Geometry check sheet. Reference: the model listing, model coordinates, mm. A direction names the side the tool comes from. Round coordinates to 2 decimals unless told otherwise and drop trailing zeros. Order: outer loops, then holes, each group sorted by start corner. A loop starts at its lowest first (then second) coordinate and runs counter-clockwise, first axis right, second up. Notation, with made-up numbers: (76, 77.25) - (117, 77.25) arc R28 ccw to (117, 98.25) - close; hole circle Ø1 at (80.5, -28). An arc over 180 degrees is marked (long way). One line per question, with ' | ' between items. Start each with the question number.
Q1. Sectioned sample at A-A, the plane z = 3.25. Enter the section's corners in (x, y), then the cut area to 3 significant figures.
Q2. Sectioned sample at D-D, the plane z = 4.75. Enter the section's corners in (x, y), then the cut area to 3 significant figures.
Q3. Gauge pin test, flat ends, axial feed: P1, Ø6, axis at x = 6.5, y = 0, coming from the +Z side; P2, Ø3, axis at y = 3.5, z = 2, coming from the -X side; P3, Ø1, axis at x = 1.5, y = -4, coming from the +Z side; P4, Ø2.5, axis at x = -6.4, y = 0, coming from the -Z side. Record the tip position at first contact, or that the pin passes through.
Q4. Tool access check on faces 1 (the face through (0, -5.2, 2)), 2 (the face through (-1, -3.7, 6)), 3 (the face through (-2.746, -4, 5)), 4 (the face through (4, -4, 3.9)), 5 (the face through (10.1, 0.1, 2)). Record the directions out of +Z, -Z, +X, -X, +Y, -Y that give a thin tool (end or side, any length) a straight path to the whole face; none if there is none.
Q5. Sectioned sample at C-C, the plane x = 3. Enter the section's corners in (y, z), then the cut area to 3 significant figures.
Q6. Material ranges on line 1 along Y through (x, z) = (-6.4, 3.6); line 2 along Y through (x, z) = (6.4, 0.8); line 3 along Z through (x, y) = (-0.5, -4.25), recorded low to high.
Q7. Sectioned sample at B-B, the plane y = 0. Enter the section's corners in (x, z).
Q8. Mould release check, pull along Y, two halves, no side actions. Record for faces 6 (the face through (-4.746, 4, 5)), 7 (the face through (11.6, -0.1, 1.2)), 8 (the face through (3, 0, 1.5)): +Y half, -Y half, draft (parallel to the pull), parting line (faces both ways), or undercut.
```python
from build123d import *

# Parameters (mm, degrees)
F1_DEPTH  = 1.5
F3_DEPTH  = 4
F4_DEPTH  = 1
F6_DEPTH  = 2.6
F7_R      = 1.6
F7_R_2    = 2.75
F8_DEPTH  = 1.501
F10_DEPTH = 5
F11_W     = 2
F11_H     = 1.5
F12_DEPTH = 1.4
F13_W     = 2
F13_H     = 1.5
F14_DEPTH = 1.4


with BuildPart() as f1:
    # F0 (on Top) → F1 (new body)
    with BuildSketch(Plane.XY):
        with BuildLine():
            Line((6.4, 5.2), (-6.4, 5.2))
            ThreePointArc((-6.4, 5.2), (-11.6, 0), (-6.4, -5.2))
            Line((-6.4, -5.2), (6.4, -5.2))
            ThreePointArc((6.4, -5.2), (11.6, 0), (6.4, 5.2))
        make_face()
    extrude(amount=F1_DEPTH)

    # F2 (on face) → F3 (join)
    with BuildSketch(Plane.XY.offset(1.5)):
        with BuildLine():
            Line((0, 5.2), (-6.4, 5.2))
            ThreePointArc((-6.4, 5.2), (-11.6, 0), (-6.4, -5.2))
            Line((-6.4, -5.2), (0, -5.2))
            Line((0, -5.2), (0, -3.7))
            Line((0, -3.7), (-6.4, -3.7))
            ThreePointArc((-6.4, -3.7), (-10.1, 0), (-6.4, 3.7))
            Line((-6.4, 3.7), (0, 3.7))
            Line((0, 3.7), (0, 5.2))
        make_face()
    extrude(amount=F3_DEPTH)

    # F2 (on face) → F4 (join)
    with BuildSketch(Plane.XY.offset(1.5)):
        with BuildLine():
            Line((6.4, 5.2), (0, 5.2))
            Line((0, 5.2), (0, 3.7))
            Line((0, 3.7), (6.4, 3.7))
            ThreePointArc((6.4, 3.7), (10.1, 0), (6.4, -3.7))
            Line((6.4, -3.7), (0, -3.7))
            Line((0, -3.7), (0, -5.2))
            Line((0, -5.2), (6.4, -5.2))
            ThreePointArc((6.4, -5.2), (11.6, 0), (6.4, 5.2))
        make_face()
    extrude(amount=F4_DEPTH)

    # F5 (on face) → F6 (join)
    with BuildSketch(Plane.XY.offset(1.5)):
        with BuildLine():
            Line((-6.4, -3.7), (-2.746235, -3.7))
            ThreePointArc((-2.746235, -3.7), (-1.2, 0), (-2.746235, 3.7))
            Line((-2.746235, 3.7), (-6.4, 3.7))
            ThreePointArc((-6.4, 3.7), (-2.7, 0), (-6.4, -3.7))
        make_face()
    extrude(amount=F6_DEPTH)

    # F7 (on face) → F8 (cut, through all)
    with BuildSketch(Plane.XY.offset(1.5)):
        with Locations((-6.4, 0)):
            Circle(F7_R)
        with Locations((6.4, 0)):
            Circle(F7_R_2)
    extrude(amount=-F8_DEPTH, mode=Mode.SUBTRACT)

    # F9 (on face) → F10 (join)
    with BuildSketch(Plane.XY.offset(1.5)):
        with BuildLine():
            Line((-2.746235, -3.7), (0, -3.7))
            Line((0, -3.7), (0, 3.7))
            Line((0, 3.7), (-2.746235, 3.7))
            ThreePointArc((-2.746235, 3.7), (-1.2, 0), (-2.746235, -3.7))
        make_face()
    extrude(amount=F10_DEPTH)

    # F11 (on face) → F12 (cut, through all)
    with BuildSketch(Plane.XY.offset(5.5)):
        with Locations((-3.746235, -4.45)):
            Rectangle(F11_W, F11_H)
        with Locations((-3.746235, 4.45)):
            Rectangle(F11_W, F11_H)
    extrude(amount=-F12_DEPTH, mode=Mode.SUBTRACT)

    # F13 (on face) → F14 (join)
    with BuildSketch(Plane.XY.offset(2.5)):
        with Locations((3.746235, -4.45)):
            Rectangle(F13_W, F13_H)
    extrude(amount=F14_DEPTH)


solid = f1.part
```
Determined:
1) outline: (-6.4, -5.2) - (0, -5.2) - (0, 5.2) - (-6.4, 5.2) arc R5.2 ccw to start; (2.75, -5.2) - (4.75, -5.2) - (4.75, -3.7) - (2.75, -3.7) - close; hole circle Ø7.4 at (-6.4, 0) | area: 69.0 mm2
2) outline: (-6.4, -5.2) - (-4.75, -5.2) - (-4.75, -3.7) - (-6.4, -3.7) arc R3.7 cw to (-6.4, 3.7) - (-4.75, 3.7) - (-4.75, 5.2) - (-6.4, 5.2) arc R5.2 ccw to start; (-2.75, -5.2) - (0, -5.2) - (0, 5.2) - (-2.75, 5.2) - (-2.75, 3.7) arc R5.2 cw to (-2.75, -3.7) - close | area: 46.6 mm2
3) P1: stops at z = 1.5 | P2: stops at x = -11.2 | P3: stops at z = 2.5 | P4: passes through
4) face 1: +Z, -Z, +X, -X, -Y | face 2: +Z, +X, -X, -Y | face 3: +Z, +Y, -Y | face 4: +Z, +X, +Y, -Y | face 5: +Z
5) outline: (-5.2, 0) - (5.2, 0) - (5.2, 2.5) - (3.7, 2.5) - (3.7, 1.5) - (-3.7, 1.5) - (-3.7, 3.9) - (-5.2, 3.9) - close | area: 20.7 mm2
6) line 1: y = -5.2 to -3.7, 3.7 to 5.2 | line 2: y = -5.2 to -2.75, 2.75 to 5.2 | line 3: z = 0 to 5.5
7) outline: (-11.6, 0) - (-8, 0) - (-8, 1.5) - (-10.1, 1.5) - (-10.1, 5.5) - (-11.6, 5.5) - close; (-4.8, 0) - (3.65, 0) - (3.65, 1.5) - (0, 1.5) - (0, 6.5) - (-1.2, 6.5) - (-1.2, 4.1) - (-2.7, 4.1) - (-2.7, 1.5) - (-4.8, 1.5) - close; (9.15, 0) - (11.6, 0) - (11.6, 2.5) - (10.1, 2.5) - (10.1, 1.5) - (9.15, 1.5) - close
8) face 6: draft | face 7: parting line | face 8: undercut
